Work out the finished part from the listing and answer in its coordinate system (mm). A direction names the side the tool comes from. Coordinates: 2 decimals unless noted, no trailing zeros. Order: outer loops, then holes, each group sorted by start corner. A loop starts at its lowest first (then second) coordinate and runs counter-clockwise, first axis right, second up. Notation, with made-up numbers: M 42.5,-13.75 L 74.5,-13.75 A14 ccw 74.5,5.25 Z; hole C -11.75,29.5 d9. An arc over 180 degrees is marked long. Write item = value, one per line. Start each with the question number.
Q1. Each of these flat-tipped pins is pushed along its axis until it touches: P1, Ø2, axis at y = 2.5, z = -1.5, coming from the -X side; P2, Ø2, axis at x = 3.5, y = 2.5, coming from the -Z side; P3, Ø3, axis at y = 2, z = -6, coming from the +X side. Where does it stop, or does it pass through?
Q2. Find section D-D on y = -0.4. Give the vertices of the cut face in (x, z), and give its area (3 significant figures).
Q3. A tool of negligible diameter and unlimited length cuts with its end or side. For faces 1 (the flat face through (6, -1, -7)), 2 (the cylindrical face through (9.01, -1.48, -7.51)), from which of +Z, -Z, +X, -X, +Y, -Y can it reach the whole face along a straight path? Write none if from no direction.
Q4. Straight lines are drawn through the part: line 1 along Y through (x, z) = (8.5, -3.5); line 2 along Y through (x, z) = (7, -3); line 3 along Z through (x, y) = (6.5, -0.95). For each, find the intervals that lie inside material, in ascending order.
Q5. Determine the mould class of faces 3 (the cylindrical face through (5.811, 0.394, -5.413)), 4 (the flat face through (6, -1, -8)), 5 (the flat face through (7, 0.8, -4)), 6 (the flat face through (0.3, 1.5, -4.1)) for opening direction X: released by +X, released by -X, zero draft, split by the parting line, or undercut.
Q6. Find section A-A on z = -3.75. Give the vertices of the cut face in (x, y), and give its area (3 significant figures).
Q7. Find section B-B on y = 0.55. Give the vertices of the cut face in (x, z), and give its area (3 significant figures).
Q8. Find section C-C on x = 4. Give the vertices of the cut face in (y, z).
```python
from build123d import *

# Parameters (mm, degrees)
SKETCH1_W               = 13
SKETCH1_H               = 8
BOSS_EXTRUDE1_DEPTH     = 3
CUT_EXTRUDE1_DEPTH      = 16.556349186
CUT_EXTRUDE1_DEPTH_BACK = 16.556349186
CUT_EXTRUDE2_DEPTH      = 16.556349186
CUT_EXTRUDE2_DEPTH_BACK = 16.556349186
SKETCH4_R               = 1.8
CUT_EXTRUDE3_DEPTH      = 0.8
SKETCH5_W               = 8
SKETCH5_H               = 1
BOSS_EXTRUDE2_DEPTH     = 2
FILLET1_R               = 4


with BuildPart() as part:
    # Sketch1 → Boss-Extrude1 (new body)
    with BuildSketch(Plane(origin=(0, 0, 0), x_dir=(1, 0, 0), z_dir=(0, 1, 0))):
        with Locations((6.5, 4)):
            Rectangle(SKETCH1_W, SKETCH1_H)
    extrude(amount=BOSS_EXTRUDE1_DEPTH)

    # Sketch2 → Cut-Extrude1 (cut, two sides: drawn at the far end of the back side and taken through both)
    with BuildSketch(Plane.XY.offset(-CUT_EXTRUDE1_DEPTH_BACK)):
        Polygon((0, 0), (0.6, 3), (0, 3), align=None)
        Polygon((13, 0), (12.4, 3), (13, 3), align=None)
    extrude(amount=CUT_EXTRUDE1_DEPTH + CUT_EXTRUDE1_DEPTH_BACK, mode=Mode.SUBTRACT)

    # Sketch3 → Cut-Extrude2 (cut, two sides: drawn at the far end of the back side and taken through both)
    with BuildSketch(Plane(origin=(0, 0, 0), x_dir=(0, 0, -1), z_dir=(1, 0, 0)).offset(-CUT_EXTRUDE2_DEPTH_BACK)):
        Polygon((0, 0), (0.6, 3), (0, 3), align=None)
        Polygon((8, 3), (7.4, 3), (8, 0), align=None)
    extrude(amount=CUT_EXTRUDE2_DEPTH + CUT_EXTRUDE2_DEPTH_BACK, mode=Mode.SUBTRACT)

    # Sketch4 → Cut-Extrude3 (cut)
    with BuildSketch(Plane.XZ):
        with Locations(Location((6.50000125, -3.75, 0), (0, 0, 270))):
            Circle(SKETCH4_R)
    extrude(amount=-CUT_EXTRUDE3_DEPTH, mode=Mode.SUBTRACT)

    # Sketch5 → Boss-Extrude2 (add)
    with BuildSketch(Plane.XZ):
        with Locations((6.500011, -7.5)):
            Rectangle(SKETCH5_W, SKETCH5_H)
    extrude(amount=BOSS_EXTRUDE2_DEPTH)

    # Fillet1
    # the kernel refuses this fillet: 4 mm, written as the material it takes off along each edge
    with BuildSketch(Plane(origin=(10.500011, -2, -16.660254038), x_dir=(0, 1, 0), z_dir=(0, 0, 1)), Plane(origin=(2.500011, -2, 1.660254038), x_dir=(0, 1, 0), z_dir=(0, 0, -1))) as fillet1_piece_1:
        with BuildLine():
            CenterArc((4, 3.464101615), FILLET1_R, 180, 60)
            Line((0, 3.464101615), (-0.08, 3.464101615))
            Line((-0.08, 3.464101615), (-0.08, 0))
            Line((-0.08, 0), (0, -0.08))
            ThreePointArc((0, -0.08), (1, -0.08), (1.96, -0.069282032))
            Line((1.96, -0.069282032), (2, 0))
        make_face()
    extrude(amount=18.320508076, mode=Mode.SUBTRACT)


solid = part.part
```
Findings below:
q1.P1 = 0.3
q1.P2 = -7.7
q1.P3 = 12.9
q2.outline = M 2.76,-8 L 10.24,-8 L 10.24,-7 L 2.76,-7 Z
q2.area = 7.47 mm^2
q3.face_1 = +Z, +X, -X, -Y
q3.face_2 = +Z, -Z, +X, -Y
q4.line_1 = 0 to 3
q4.line_2 = 0.8 to 3
q4.line_3 = -8 to -7
q5.face_3 = undercut
q5.face_4 = zero draft
q5.face_5 = undercut
q5.face_6 = released by -X
q6.outline = M 0,0 L 4.7,0 L 4.7,0.8 L 8.3,0.8 L 8.3,0 L 13,0 L 12.4,3 L 0.6,3 Z
q6.area = 34.3 mm^2
q7.outline = M 0.11,-7.89 L 12.89,-7.89 L 12.89,-0.11 L 0.11,-0.11 Z; hole C 6.5,-3.75 d3.6
q7.area = 89.2 mm^2
q8.outline = M -1.48,-8 L 0,-8 L 3,-7.4 L 3,-0.6 L 0,0 L 0,-7 L -1.48,-7 Z
